Model file for the job. Use its own axes, mm. Face numbers are marked on the shaded views. A direction names the side the tool comes from. Round coordinates to 2 decimals unless told otherwise and drop trailing zeros. Order: outer loops, then holes, each group sorted by start corner. A loop starts at its lowest first (then second) coordinate and runs counter-clockwise, first axis right, second up. Notation, with made-up numbers: (2, 37.25) - (41, 37.25) arc R28 ccw to (41, 70.25) - close; hole circle Ø10 at (27.5, 19). An arc over 180 degrees is marked (long way). Use one line per item in the form item = value.
from build123d import *

# Parameters (mm, degrees)
SKETCH1_R               = 9
BOSS_EXTRUDE1_DEPTH     = 15
BOSS_EXTRUDE2_START     = 10
BOSS_EXTRUDE2_DEPTH     = 10
DOME2_FACE_RADIUS       = 9
DOME2_HEIGHT            = 5
CUT_EXTRUDE1_DEPTH      = 24.706539182
CUT_EXTRUDE1_DEPTH_BACK = 24.706539182
SKETCH3_R               = 1.5
FILLET4_R               = 10
CUT_EXTRUDE2_DEPTH      = 24.706539182
CUT_EXTRUDE2_DEPTH_BACK = 24.706539182
SKETCH4_R               = 0.625
SKETCH5_W               = 3
SKETCH5_H               = 2
CUT_EXTRUDE3_DEPTH      = 20
SKETCH6_R               = 0.9
CUT_EXTRUDE4_DEPTH      = 5


with BuildPart() as part:
    # Sketch1 → Boss-Extrude1 (new body)
    with BuildSketch(Plane.XY):
        Circle(SKETCH1_R)
    extrude(amount=-BOSS_EXTRUDE1_DEPTH)

    # Sketch2 → Boss-Extrude2 (add)
    with BuildSketch(Plane.XY.offset(BOSS_EXTRUDE2_START)):
        with BuildLine():
            Line((-4.5, 7.794228634), (-4.5, -7.794228634))
            ThreePointArc((-4.5, -7.794228634), (0, -9), (4.5, -7.794228634))
            Line((4.5, -7.794228634), (4.5, 7.794228634))
            Line((4.5, 7.794228634), (-4.5, 7.794228634))
        make_face()
    extrude(amount=-BOSS_EXTRUDE2_DEPTH)

    # Dome2: a dome of height H over a round flat face of radius A is a cap of a sphere of radius (A * A + H * H) / (2 * H)
    dome2_r = (DOME2_FACE_RADIUS * DOME2_FACE_RADIUS + DOME2_HEIGHT * DOME2_HEIGHT) / (2 * DOME2_HEIGHT)
    dome2_base = Plane((0, 0, -15), z_dir=(0, 0, -1))
    with Locations(dome2_base.offset(DOME2_HEIGHT - dome2_r)):
        dome2_ball = Sphere(dome2_r, mode=Mode.PRIVATE)
    add(split(dome2_ball, bisect_by=dome2_base, keep=Keep.TOP, mode=Mode.PRIVATE))

    # Sketch3 → Cut-Extrude1 (cut, two sides: drawn at the far end of the back side and taken through both)
    with BuildSketch(Plane(origin=(0, 0, 0), x_dir=(0, 0, -1), z_dir=(1, 0, 0)).offset(-CUT_EXTRUDE1_DEPTH_BACK)):
        with Locations((-5, 0)):
            Circle(SKETCH3_R)
    extrude(amount=CUT_EXTRUDE1_DEPTH + CUT_EXTRUDE1_DEPTH_BACK, mode=Mode.SUBTRACT)

    # Fillet4
    fillet4_edges = [part.edges().sort_by_distance(p)[0] for p in [
        (0, 7.794228634, 10),
    ]]
    fillet(fillet4_edges, radius=FILLET4_R - 0.0001)  # a hair under: the kernel refuses the full size

    # Sketch4 → Cut-Extrude2 (cut, two sides: drawn at the far end of the back side and taken through both)
    with BuildSketch(Plane.XY.offset(-CUT_EXTRUDE2_DEPTH_BACK)):
        with Locations(Location((0, 7.5, 0), (0, 0, 28.084018699))):
            Circle(SKETCH4_R)
    extrude(amount=CUT_EXTRUDE2_DEPTH + CUT_EXTRUDE2_DEPTH_BACK, mode=Mode.SUBTRACT)

    # Sketch5 → Cut-Extrude3 (cut)
    with BuildSketch(Plane.XY.offset(10)):
        with Locations((0, -9)):
            Rectangle(SKETCH5_W, SKETCH5_H)
    extrude(amount=-CUT_EXTRUDE3_DEPTH, mode=Mode.SUBTRACT)

    # Sketch6 → Cut-Extrude4 (cut)
    with BuildSketch(Plane(origin=(0, -8, 0), x_dir=(-1, 0, 0), z_dir=(0, -1, 0))):
        with Locations(Location((0, 7, 0), (0, 0, 90))):
            Circle(SKETCH6_R)
    extrude(amount=-CUT_EXTRUDE4_DEPTH, mode=Mode.SUBTRACT)


solid = part.part
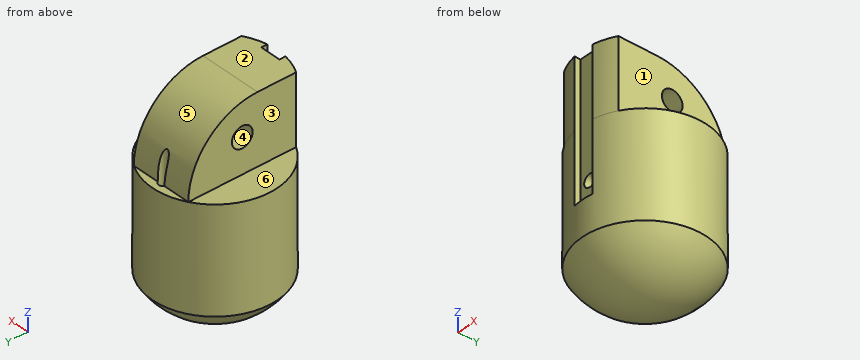
(1) Tool access for the marked faces 1, 2 and 3: list every direction of +Z, -Z, +X, -X, +Y, -Y with a clear straight run to the whole face (end or side of a thin tool).
Report:
face_1 = +Z, +X, +Y, -Y
face_2 = +Z, +X, -X, +Y, -Y
face_3 = +Z, -X, +Y, -Y
(2) Slice it at B-B on x = 0. Give the cut face in (y, z) (3 decimals), then the cut area to 3 significant figures.
Report:
outline = (-9, -15) arc R10.6 ccw to (6.875, -17.468) - (6.875, 4.188) arc R10 ccw to (-2.206, 10) - (-8, 10) - (-8, -6.1) - (-3, -6.1) - (-3, -7.9) - (-8, -7.9) - (-8, -10) - (-9, -10) - close; (8.125, -16.208) arc R10.6 ccw to (9, -15) - (9, 0) - (8.125, 0) - close; hole circle Ø3 at (0, 5)
area = 420 mm2
(3) Slice it at C-C on y = 0. Give the cut face in (x, z).
Report:
outline = (-9, -15) arc R10.6 ccw to (9, -15) - (9, 0) - (4.5, 0) - (4.5, 3.5) - (-4.5, 3.5) - (-4.5, 0) - (-9, 0) - close; (-4.5, 6.5) - (4.5, 6.5) - (4.5, 9.75) - (-4.5, 9.75) - close
(4) Probe probe 1 along Y at (x, z) = (0, -1.25) (3 decimals); probe 2 along Y at (x, z) = (0, -12.5) (3 decimals); probe 3 along X at (y, z) = (2.75, 4.5). List the from-to ranges inside material, lowest first. Write a range as [from, to].
Report:
probe_1 = [-8, 6.875], [8.125, 9]
probe_2 = [-9, 6.875], [8.125, 9]
probe_3 = [-4.5, 4.5]
(5) Slice it at D-D on z = 5. Give the cut face in (x, y).
Report:
outline = (-4.5, -7.79) arc R9 ccw to (-1.5, -8.87) - (-1.5, -8) - (1.5, -8) - (1.5, -8.87) arc R9 ccw to (4.5, -7.79) - (4.5, -1.5) - (-4.5, -1.5) - close; (-4.5, 1.5) - (4.5, 1.5) - (4.5, 6.45) - (-4.5, 6.45) - close
(6) Slice it at A-A on z = -7. Give the cut face in (x, y) (3 decimals), then the cut area to 3 significant figures.
Report:
outline = (-1.5, -8.874) - (-1.5, -8) - (-0.9, -8) - (-0.9, -3) - (0.9, -3) - (0.9, -8) - (1.5, -8) - (1.5, -8.874) arc R9 ccw (long way) to start; hole circle Ø1.25 at (0, 7.5)
area = 241 mm2
(7) Pull direction Y, two halves, no side cores. Call the marked faces 4, 5 and 6: released by +Y, released by -Y, zero draft, split by the parting line, or undercut.
Report:
face_4 = undercut
face_5 = released by +Y
face_6 = zero draft
(8) Pin check, flat tips, straight feed: pin 1 (1 mm diameter, centred on y = -8.5, z = 4, fed in from +X); pin 2 (0.9 mm diameter, centred on x = 0, z = -4, fed in from -Y); pin 3 (2 mm diameter, centred on x = -7, y = 3.5, fed in from -Z); pin 4 (2 mm diameter, centred on x = 7, z = 6, fed in from +Y). Stop position of each tip, or through.
Report:
pin_1 = 4.12
pin_2 = -8
pin_3 = -17.51
pin_4 = through
